```python
from build123d import *

# Parameters (mm, degrees)
ANGLES_EQUAL_50_X_50_X_3_1_DEPTH = 98
F_18_0_18_DIAMETER_HOLE1_D       = 18
LPATTERN1_COUNT                  = 2
LPATTERN1_PITCH                  = 50


with BuildPart() as part:
    # Sketch14 → Angles equal 50 X 50 X 3(1) (new body)
    with BuildSketch(Plane(origin=(0, 25, 25), x_dir=(0, 1, 0), z_dir=(1, 0, 0))):
        with BuildLine():
            Line((-25, 25), (-25, -25))
            Line((-25, -25), (25, -25))
            Line((25, -25), (25, -24.5))
            ThreePointArc((25, -24.5), (24.267766953, -22.732233047), (22.5, -22))
            Line((22.5, -22), (-15, -22))
            ThreePointArc((-15, -22), (-19.949747468, -19.949747468), (-22, -15))
            Line((-22, -15), (-22, 22.5))
            ThreePointArc((-22, 22.5), (-22.732233047, 24.267766953), (-24.5, 25))
            Line((-24.5, 25), (-25, 25))
        make_face()
    extrude(amount=ANGLES_EQUAL_50_X_50_X_3_1_DEPTH)

    # Ø18.0 (18) Diameter Hole1 (through all)
    with Locations(Plane(origin=(0, 3, 0), x_dir=(1, 0, 0), z_dir=(0, 1, 0))):
        with Locations((24, -28)):
            f_18_0_18_diameter_hole1 = Hole(F_18_0_18_DIAMETER_HOLE1_D / 2)

    # LPattern1: Ø18.0 (18) Diameter Hole1 ×2
    with Locations(*[(i * LPATTERN1_PITCH, 0, 0) for i in range(1, LPATTERN1_COUNT)]):
        add(f_18_0_18_diameter_hole1, mode=Mode.SUBTRACT)


solid = part.part
```
Verification items for the finished model (mm, model axes). A direction names the side the tool comes from. Coordinates: 2 decimals unless noted, no trailing zeros. Loops run counter-clockwise (first coordinate to the right, second up) from the corner with the lowest first, then second, coordinate; pieces in that order, holes last. Notation, with made-up numbers: (40, 81) - (53, 81) arc R23 cw to (53, 91) - close; hole circle Ø4 at (12, -26.75). An arc over 180 degrees is marked (long way). Return JSON: item names as keys, results as strings.
1. Section check D-D, the plane z = 44. Record the boundary of the cut face in (x, y), then the cut area to 3 significant figures.
Established:
{"outline": "(0, 0) - (98, 0) - (98, 3) - (0, 3) - close", "area": "294 mm2"}
2. Section check C-C, the plane x = 54. Record the boundary of the cut face in (y, z), then the cut area to 3 significant figures.
Established:
{"outline": "(0, 0) - (50, 0) - (50, 0.5) arc R2.5 ccw to (47.5, 3) - (10, 3) arc R7 cw to (3, 10) - (3, 47.5) arc R2.5 ccw to (0.5, 50) - (0, 50) - close", "area": "299 mm2"}
3. Tool access check on faces 1 (the flat face through (48, 29, 3)), 2 (the cylindrical face through (19.16, 1.48, 20.41)). Record the directions out of +Z, -Z, +X, -X, +Y, -Y that give a thin tool (end or side, any length) a straight path to the whole face; none if there is none.
Established:
{"face 1": "+Z, +X, -X, +Y", "face 2": "+Y, -Y"}
4. Section check A-A, the plane z = 28. Record the boundary of the cut face in (x, y), then the cut area to 3 significant figures.
Established:
{"outline": "(0, 0) - (15, 0) - (15, 3) - (0, 3) - close; (33, 0) - (65, 0) - (65, 3) - (33, 3) - close; (83, 0) - (98, 0) - (98, 3) - (83, 3) - close", "area": "186 mm2"}
5. Mould release check, pull along Z, two halves, no side actions. Record for faces 3 (the flat face through (48, 3, 28)), 4 (the cylindrical face through (65.416, 1.479, 25.297)), 5 (the cylindrical face through (48.314, 2.287, 49.248)): +Z half, -Z half, draft (parallel to the pull), parting line (faces both ways), or undercut.
Established:
{"face 3": "draft", "face 4": "undercut", "face 5": "+Z half"}
6. Thickness scan on L1, parallel to Z at x = 30, y = 47; L2, parallel to Z at x = 24, y = 0.95. Record the ranges inside material, lowest first.
Established:
{"L1": "z = 0 to 3", "L2": "z = 0 to 19, 37 to 49.96"}
7. Section check B-B, the plane x = 74. Record the boundary of the cut face in (y, z).
Established:
{"outline": "(0, 0) - (50, 0) - (50, 0.5) arc R2.5 ccw to (47.5, 3) - (10, 3) arc R7 cw to (3, 10) - (3, 19) - (0, 19) - close; (0, 37) - (3, 37) - (3, 47.5) arc R2.5 ccw to (0.5, 50) - (0, 50) - close"}
8. Go/stop test with flat-tipped pins: pin 1 (10 mm diameter, centred on x = 24.5, y = 16, fed in from +Z); pin 2 (20.5 mm diameter, centred on x = 74, z = 28, fed in from +Y). Record where each tip stops, or that it passes through.
Established:
{"pin 1": "stops at z = 3", "pin 2": "stops at y = 3"}
